Check sheet for the modelled part. Datum: model origin and axes. Units: mm. Round coordinates to 2 decimals unless told otherwise and drop trailing zeros. Order: outer loops, then holes, each group sorted by start corner. A loop starts at its lowest first (then second) coordinate and runs counter-clockwise, first axis right, second up. Notation, with made-up numbers: (31.5, 50.5) -> (82.5, 50.5) arc R6 cw to (82.5, 55.5) -> close; hole circle Ø4 at (70, 28.5). An arc over 180 degrees is marked (long way). Answer in a Markdown table with one row per item. Add a question column.
1. Material ranges on L1, parallel to Z at x = 0, y = 1.35; L2, parallel to X at y = 0.3, z = 43.5; L3, parallel to X at y = 1.05, z = 63.5, recorded low to high. Write a range as from..to.
2. Sectioned sample at B-B, the plane z = 42. Record the boundary of the cut face in (x, y), then the cut area to 3 significant figures.
3. Sectioned sample at A-A, the plane x = 0. Record the boundary of the cut face in (y, z), then the cut area to 3 significant figures.
4. Depth check by flat-ended pin: P1, Ø0.5, axis at x = 0.5, y = 0, coming from the +Z side; P2, Ø1.5, axis at x = -1, z = 9, coming from the -Y side. Enter the tip coordinate at first touch or a pass-through.
```python
from build123d import *

# Parameters (mm, degrees)
F0_R     = 1.5
F1_DEPTH = 65
F3_DEPTH = 4
F4_R     = 0.5
F5_DEPTH = 1.5
F6_R     = 0.5


with BuildPart() as f1:
    # F0 (on Top) → F1 (new body)
    with BuildSketch(Plane.XY):
        Circle(F0_R)
    extrude(amount=F1_DEPTH)

    # F2 (on face) → F3 (cut)
    with BuildSketch(Plane.XY.offset(65)):
        with BuildLine():
            Line((1.268857754, 0.8), (-1.268857754, 0.8))
            ThreePointArc((-1.268857754, 0.8), (-1.5, 0), (-1.268857754, -0.8))
            Line((-1.268857754, -0.8), (1.268857754, -0.8))
            ThreePointArc((1.268857754, -0.8), (1.4410563193, -0.4163612428), (1.5, 0))
            ThreePointArc((1.5, 0), (1.4410563193, 0.4163612428), (1.268857754, 0.8))
        make_face()
    extrude(amount=-F3_DEPTH, mode=Mode.SUBTRACT)

    # F4 (on Front) → F5 (cut, symmetric)
    with BuildSketch(Plane.XZ):
        with Locations((0, 63.5)):
            Circle(F4_R)
    extrude(amount=F5_DEPTH, both=True, mode=Mode.SUBTRACT)

    # F6
    f6_edges = [f1.edges().sort_by_distance(p)[0] for p in [
        (0, -0.8, 61),
        (0, 0.8, 61),
    ]]
    fillet(f6_edges, radius=F6_R)


solid = f1.part
```
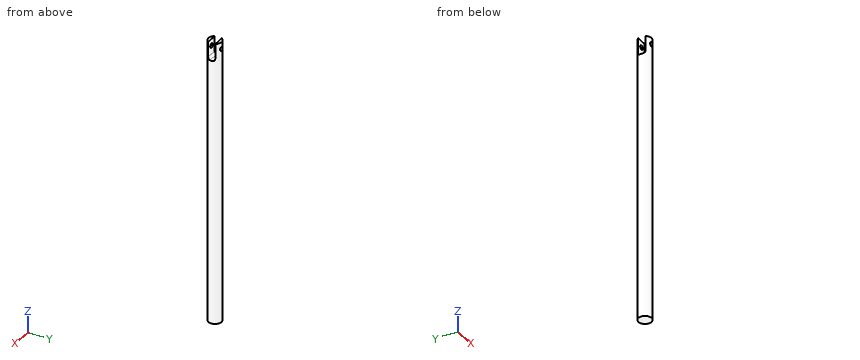
Answer key:
| question | item | result |
|---|---|---|
| 1 | L1 | z = 0..63, 64..65 |
| 1 | L2 | x = -1.47..1.47 |
| 1 | L3 | x = -1.07..-0.5, 0.5..1.07 |
| 2 | outline | circle Ø3 at (0, 0) |
| 2 | area | 7.07 mm² |
| 3 | outline | (-1.5, 0) -> (1.5, 0) -> (1.5, 63) -> (0.8, 63) -> (0.8, 61.5) arc R0.5 cw to (0.3, 61) -> (-0.3, 61) arc R0.5 cw to (-0.8, 61.5) -> (-0.8, 63) -> (-1.5, 63) -> close; (-1.5, 64) -> (-0.8, 64) -> (-0.8, 65) -> (-1.5, 65) -> close; (0.8, 64) -> (1.5, 64) -> (1.5, 65) -> (0.8, 65) -> close |
| 3 | area | 187 mm² |
| 4 | P1 | stops at z = 61 |
| 4 | P2 | stops at y = -1.48 |
